Build history of the part. All positions in model axes, mm. A direction names the side the tool comes from. Give positions to 0.01 mm unless a question says otherwise; leave off trailing zeros. Loops run counter-clockwise (first coordinate to the right, second up) from the corner with the lowest first, then second, coordinate; pieces in that order, holes last. Notation, with made-up numbers: (-27, 55.25) -> (17, 55.25) arc R11 ccw to (17, 76.25) -> close; hole circle Ø5 at (57.25, -20.75). An arc over 180 degrees is marked (long way). One line per question, with ' | ' between items. Start each with the question number.
(1) Flat gauge pins, fed straight in: pin 1 Ø2.5 at (x, y) = (-15.5, 16) entering from +Z; pin 2 Ø2.5 at (x, y) = (15.5, 15.5) entering from +Z; pin 3 Ø6 at (x, z) = (-3, -7.5) entering from -Y; pin 4 Ø8 at (y, z) = (-4.5, -0.5) entering from -X. Where does each tip first touch, or does it go through?
(2) 3-axis set-ups, long thin cutter, end or side, ignore diameter. For faces 1 (the face through (0, 19.15, -10)), 2 (the face through (14, 15.57, 7.78)), 3 (the face through (2, -20, -20)), 4 (the face through (-19.2, 19.1, -24.9)): which of +Z, -Z, +X, -X, +Y, -Y reach the whole face in a straight line?
(3) Slice it at C-C, the plane y = 9.5. Write the cut outline in (x, z).
(4) Drill centre lines: L1, parallel to Y at x = 15.5, z = 7.25; L2, parallel to Z at x = 13.5, y = 13; L3, parallel to Z at x = 14.5, y = 16. Where is each one in solid material? Low to high. Write a range as from..to.
(5) Slice it at A-A, the plane x = 0. Write the cut outline in (y, z), then the cut area to 3 significant figures.
(6) Mould opens along Z. For faces 5 (the face through (19.15, 0, -10)), 6 (the face through (0, 21.15, -25)), 7 (the face through (-16, 16, 5.5)) say: pulls with the +Z half, pulls with the -Z half, needs draft (parallel to the pull), parting line crosses it, or undercut.
(7) Slice it at B-B, the plane z = 7. Write the cut outline in (x, y).
(8) Slice it at D-D, the plane y = -15.5. Write the cut outline in (x, z), then the cut area to 4 significant figures.
```python
from build123d import *

# Parameters (mm, degrees)
BOSS_EXTRUDE1_DEPTH = 10
BOSS_EXTRUDE2_DEPTH = 20
BOSS_EXTRUDE3_DEPTH = 10
BOSS_EXTRUDE4_DEPTH = 22
SKETCH6_R           = 1.5
CUT_EXTRUDE1_DEPTH  = 4.5


with BuildPart() as part:
    # Sketch1 → Boss-Extrude1 (new body)
    with BuildSketch(Plane.XY):
        Polygon((-21.15, 17.15), (-17.15, 21.15), (17.15, 21.15), (21.15, 17.15), (21.15, -17.15), (17.15, -21.15), (-17.15, -21.15), (-21.15, -17.15), align=None)
    extrude(amount=BOSS_EXTRUDE1_DEPTH)

    # Sketch2 → Boss-Extrude2 (add)
    with BuildSketch(Plane(origin=(0, 0, 0), x_dir=(-1, 0, 0), z_dir=(0, 0, -1))):
        Polygon((19.15, 16.321572875), (16.321572875, 19.15), (-16.321572875, 19.15), (-19.15, 16.321572875), (-19.15, -16.321572875), (-16.321572875, -19.15), (16.321572875, -19.15), (19.15, -16.321572875), align=None)
    extrude(amount=BOSS_EXTRUDE2_DEPTH)

    # Sketch3 → Boss-Extrude3 (add)
    with BuildSketch(Plane(origin=(0, 0, -20), x_dir=(-1, 0, 0), z_dir=(0, 0, -1))):
        Polygon((21.15, 17.15), (17.15, 21.15), (-17.15, 21.15), (-21.15, 17.15), (-21.15, -17.15), (-17.15, -21.15), (17.15, -21.15), (21.15, -17.15), align=None)
    extrude(amount=BOSS_EXTRUDE3_DEPTH)

    # Sketch4 → Boss-Extrude4 (add)
    with BuildSketch(Plane.XY.offset(10)):
        with BuildLine():
            Line((2.291287847, 1), (-2.291287847, 1))
            ThreePointArc((-2.291287847, 1), (-0.510774109, -2.447265782), (2.5, 0))
            ThreePointArc((2.5, 0), (2.447265782, 0.510774109), (2.291287847, 1))
        make_face()
    extrude(amount=BOSS_EXTRUDE4_DEPTH)

    # Sketch6 → Cut-Extrude1 (cut)
    with BuildSketch(Plane.XY.offset(10)):
        with Locations((-15.5, 15.5)):
            Circle(SKETCH6_R)
        with Locations((15.5, 15.5)):
            Circle(SKETCH6_R)
        with Locations((15.5, -15.5)):
            Circle(SKETCH6_R)
        with Locations((-15.5, -15.5)):
            Circle(SKETCH6_R)
    extrude(amount=-CUT_EXTRUDE1_DEPTH, mode=Mode.SUBTRACT)


solid = part.part
```
Final values:
1) pin 1: z = 10 | pin 2: z = 5.5 | pin 3: y = -19.15 | pin 4: x = -21.15
2) face 1: +X, -X, +Y | face 2: +Z | face 3: none | face 4: +Z, -Z, -X, +Y
3) outline: (-21.15, -30) -> (21.15, -30) -> (21.15, -20) -> (19.15, -20) -> (19.15, 0) -> (21.15, 0) -> (21.15, 10) -> (-21.15, 10) -> (-21.15, 0) -> (-19.15, 0) -> (-19.15, -20) -> (-21.15, -20) -> close
4) L1: -21.15..-17, -14..14, 17..21.15 | L2: -30..10 | L3: -30..5.5
5) outline: (-21.15, -30) -> (21.15, -30) -> (21.15, -20) -> (19.15, -20) -> (19.15, 0) -> (21.15, 0) -> (21.15, 10) -> (1, 10) -> (1, 32) -> (-2.5, 32) -> (-2.5, 10) -> (-21.15, 10) -> (-21.15, 0) -> (-19.15, 0) -> (-19.15, -20) -> (-21.15, -20) -> close | area: 1,690 mm2
6) face 5: undercut | face 6: needs draft | face 7: pulls with the +Z half
7) outline: (-21.15, -17.15) -> (-17.15, -21.15) -> (17.15, -21.15) -> (21.15, -17.15) -> (21.15, 17.15) -> (17.15, 21.15) -> (-17.15, 21.15) -> (-21.15, 17.15) -> close; hole circle Ø3 at (-15.5, -15.5); hole circle Ø3 at (-15.5, 15.5); hole circle Ø3 at (15.5, -15.5); hole circle Ø3 at (15.5, 15.5)
8) outline: (-21.15, -30) -> (21.15, -30) -> (21.15, -20) -> (19.15, -20) -> (19.15, 0) -> (21.15, 0) -> (21.15, 10) -> (17, 10) -> (17, 5.5) -> (14, 5.5) -> (14, 10) -> (-14, 10) -> (-14, 5.5) -> (-17, 5.5) -> (-17, 10) -> (-21.15, 10) -> (-21.15, 0) -> (-19.15, 0) -> (-19.15, -20) -> (-21.15, -20) -> close | area: 1,585 mm2
